Part model, mm, in its own coordinate system. Face numbers are marked on the shaded views. Coordinates: 2 decimals unless noted, no trailing zeros. Order: outer loops, then holes, each group sorted by start corner. A loop starts at its lowest first (then second) coordinate and runs counter-clockwise, first axis right, second up.
1) Pin check, flat tips, straight feed: pin 1 Ø7.5 at (x, y) = (108, -46.5) entering from +Z; pin 2 Ø5.5 at (x, y) = (-103.5, 48.5) entering from +Z; pin 3 Ø1.5 at (y, z) = (46, 7) entering from -X; pin 4 Ø5 at (y, z) = (-12, 2.5) entering from +X. Stop position of each tip, or through.
2) Cut at A-A (x = -13.5). List the corners of the cut face in (y, z).
3) Wall check: L1, parallel to Y at x = -85, z = 9.25; L2, parallel to Y at x = 103.5, z = 2.4; L3, parallel to X at y = 55, z = 8. Give the ranges that are in metal, low to high.
4) Mould opens along Y. For the marked faces 1 and 2 say: +Y half, -Y half, draft (parallel to the pull), parting line (faces both ways), or undercut.
5) Cut at D-D (x = 96). List the corners of the cut face in (y, z).
6) Cut at B-B (z = 10.75). List the corners of the cut face in (x, y).
7) Cut at C-C (y = 16.5). List the corners of the cut face in (x, z), and give its area (3 significant figures).
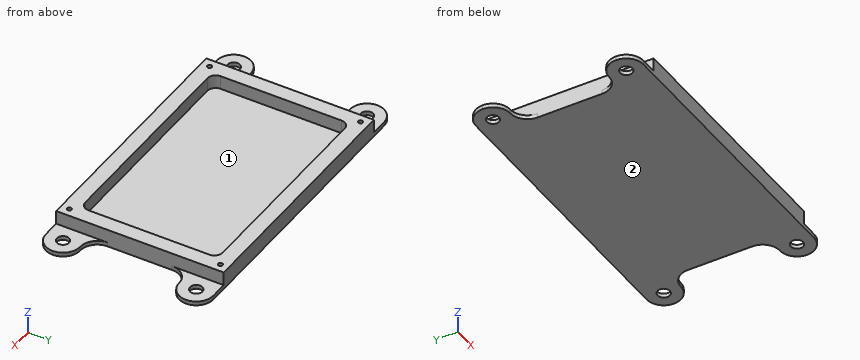
Autodesk Inventor part; units mm, degrees
ref_plane "YZ Plane" through (0, 0, 0) normal (1, 0, 0) x (0, 1, 0)
ref_plane "XZ Plane" through (0, 0, 0) normal (0, 1, 0) x (-1, 0, 0)
ref_plane "XY Plane" through (0, 0, 0) normal (0, 0, 1) x (1, 0, 0)
sketch "Sketch1" plane through (0, 0, 0) normal (0, 0, 1) x (1, 0, 0)
  line L0 (-83, 53) -> (83, 53) construction
  line L1 (83, 53) -> (83, -53) construction
  line L2 (83, -53) -> (-83, -53) construction
  line L3 (-83, -53) -> (-83, 53) construction
  line L4 (-83, -53) -> (83, 53) construction
  line L5 (83, -53) -> (-83, 53) construction
  line L6 (-91, 61) -> (91, 61)
  line L7 (91, 61) -> (91, -61)
  line L8 (91, -61) -> (-91, -61)
  line L9 (-91, -61) -> (-91, 61)
  line L10 (-91, 61) -> (91, -61) construction
  line L11 (-91, -61) -> (91, 61) construction
  line L12 (-91, 61) -> (-116, 61)
  line L13 (-116, 61) -> (-116, 36)
  line L14 (-116, 36) -> (-91, 36)
  line L15 (-91, 36) -> (-91, 61)
  line L16 (0, 0) -> (-160.1953, 0) construction
  line L17 (-91, -61) -> (-116, -61)
  line L18 (-116, -61) -> (-116, -36)
  line L19 (-116, -36) -> (-91, -36)
  line L20 (-91, -36) -> (-91, -61)
  line L21 (0, 0) -> (0, 107.5555) construction
  line L22 (91, -61) -> (91, 61)
  line L23 (91, 61) -> (116, 61)
  line L24 (116, 61) -> (116, 36)
  line L25 (116, 36) -> (91, 36)
  line L26 (91, 36) -> (91, 61)
  line L27 (91, -36) -> (91, -61)
  line L28 (91, -61) -> (116, -61)
  line L29 (116, -61) -> (116, -36)
  line L30 (116, -36) -> (91, -36)
  point P0 (0, 0)
  point P1 (0, 0)
  dimension "d0" = 166
  dimension "d1" = 106
  dimension "d2" = 8
  dimension "d3" = 8
  dimension "d4" = 25
  dimension "d5" = 25
extrude "Extrusion1" add sketch "Sketch1" along normal blind 3
sketch "Sketch2" plane through (0, 0, 3) normal (0, 0, 1) x (1, 0, 0)
  line L0 (-116, 61) -> (116, 61)
  line L1 (-116, 36) -> (-116, 61)
  line L2 (116, 61) -> (116, 36)
  circle A0 centre (-103.5, 48.5) radius 1
  line L3 (0, 0) -> (-24.3275, 0) construction
  line L4 (0, 0) -> (0, 26.5856) construction
  circle A1 centre (-103.5, -48.5) radius 1
  circle A2 centre (103.5, 48.5) radius 1
  circle A3 centre (103.5, -48.5) radius 1
  dimension "d8" = 2
  dimension "d9" = 12.5
  dimension "d10" = 12.5
hole "Hole1" at (-103.5, 48.5, 3) at (-103.5, -48.5, 3) at (103.5, -48.5, 3) at (103.5, 48.5, 3) direction (0, 0, -1) diameter 9 depth 8 tip angle 118
fillet "Fillet1" radius 12.5 12 edges at (116, 61, 1.5) (116, 36, 1.5) (91, 36, 1.5) (91, -36, 1.5) (116, -36, 1.5) (116, -61, 1.5) (-116, -61, 1.5) (-116, -36, 1.5) (-91, -36, 1.5) (-91, 36, 1.5) (-116, 36, 1.5) (-116, 61, 1.5)
sketch "Sketch3" plane through (0, 0, 3) normal (0, 0, 1) x (1, 0, 0)
  line L0 (103.5, -61) -> (-103.5, -61)
  line L1 (-103.5, 61) -> (103.5, 61)
  line L2 (-91, 61) -> (91, 61)
  line L3 (91, 61) -> (91, -61)
  line L4 (91, -61) -> (-91, -61)
  line L5 (-91, -61) -> (-91, 61)
  line L6 (-80, 50) -> (80, 50)
  line L7 (80, 50) -> (80, -50)
  line L8 (80, -50) -> (-80, -50)
  line L9 (-80, -50) -> (-80, 50)
  line L10 (-80, 50) -> (80, -50) construction
  line L11 (-80, -50) -> (80, 50) construction
  line L12 (-91, -23.5) -> (-91, 23.5)
  point P0 (0, 0)
  dimension "d19" = 100
  dimension "d20" = 160
extrude "Extrusion2" add sketch "Sketch3" along normal blind 10
fillet "Fillet2" radius 6 4 edges at (-80, 50, 8) (-80, -50, 8) (80, -50, 8) (80, 50, 8)
sketch "Sketch6" plane through (0, 0, 13) normal (0, 0, 1) x (1, 0, 0)
  line L0 (-91, 61) -> (91, 61)
  line L1 (-91, -61) -> (-91, 61)
  circle A0 centre (-85, 55) radius 2
  line L2 (0, 0) -> (-11.4122, 0) construction
  line L3 (0, 0) -> (0, 13.6861) construction
  circle A1 centre (-85, -55) radius 2
  circle A2 centre (85, 55) radius 2
  circle A3 centre (85, -55) radius 2
  dimension "d33" = 4
  dimension "d34" = 6
  dimension "d35" = 6
hole "Hole2" at (-85, 55, 13) at (-85, -55, 13) at (85, -55, 13) at (85, 55, 13) direction (0, 0, -1) diameter 3.242 depth 8 tip angle 118
equation "\"d34\" = 1.5 * d33"
equation "\"d35\" = 1.5 * d33"
properties part number "Base.Box.Base"
Geometry check:
1. pin 1: stops at z = 3
1. pin 2: passes through
1. pin 3: stops at x = -91
1. pin 4: stops at x = 91
2. outline: (-61, 0) - (61, 0) - (61, 13) - (50, 13) - (50, 3) - (-50, 3) - (-50, 13) - (-61, 13) - close
3. L1: y = -61 to -56.62, -53.38 to 53.38, 56.62 to 61
3. L2: y = -61 to -53, -44 to -36, 36 to 44, 53 to 61
3. L3: x = -91 to -86.62, -83.38 to 83.38, 86.62 to 91
4. face 1: undercut
4. face 2: draft
5. outline: (-61, 0) - (-33.5, 0) - (-33.5, 3) - (-61, 3) - close; (33.5, 0) - (61, 0) - (61, 3) - (33.5, 3) - close
6. outline: (-91, -61) - (91, -61) - (91, 61) - (-91, 61) - close; hole circle Ø3.24 at (-85, -55); hole circle Ø3.24 at (-85, 55); hole (-80, -44) arc R6 ccw to (-74, -50) - (74, -50) arc R6 ccw to (80, -44) - (80, 44) arc R6 ccw to (74, 50) - (-74, 50) arc R6 ccw to (-80, 44) - close; hole circle Ø3.24 at (85, -55); hole circle Ø3.24 at (85, 55)
7. outline: (-91, 0) - (91, 0) - (91, 13) - (80, 13) - (80, 3) - (-80, 3) - (-80, 13) - (-91, 13) - close
7. area: 766 mm2
